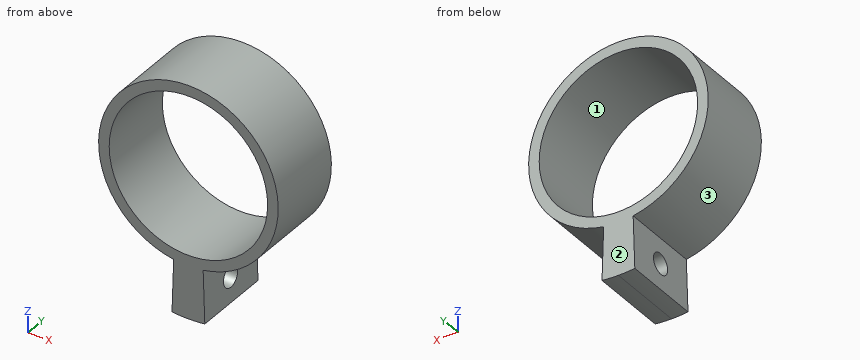
from build123d import *

# Parameters (mm, degrees)
F0_R     = 17
F0_R_2   = 15
F1_DEPTH = 15
F3_DEPTH = 15
F4_R     = 2
F5_DEPTH = 20.10135


with BuildPart() as f1:
    # F0 (on Front) → F1 (new body)
    with BuildSketch(Plane.XZ):
        Circle(F0_R)
        Circle(F0_R_2, mode=Mode.SUBTRACT)
    extrude(amount=F1_DEPTH)

    # F2 (on face) → F3 (join)
    with BuildSketch(Plane(origin=(0, 0, 0), x_dir=(-1, 0, 0), z_dir=(0, 1, 0))):
        with BuildLine():
            Line((-2.790576, -16.769397), (-3.104631, -26.764465))
            ThreePointArc((-3.104631, -26.764465), (-1.554907, -26.899025), (0, -26.943929))
            ThreePointArc((0, -26.943929), (1.554907, -26.899025), (3.104631, -26.764465))
            Line((3.104631, -26.764465), (2.790576, -16.769397))
            ThreePointArc((2.790576, -16.769397), (1.400044, -16.942251), (0, -17))
            ThreePointArc((0, -17), (-1.400044, -16.942251), (-2.790576, -16.769397))
        make_face()
    extrude(amount=-F3_DEPTH)

    # F4 (on face) → F5 (cut, through all)
    with BuildSketch(Plane(origin=(-2.261431, 0, 0.071057), x_dir=(0, -1, 0), z_dir=(-0.999507, 0, 0.031406))):
        with Locations((7.5, -21.848765)):
            Circle(F4_R)
    extrude(amount=-F5_DEPTH, mode=Mode.SUBTRACT)


solid = f1.part
Design review of the part built by this model. Coordinates are the model's own, in mm. Face numbers are marked on the shaded views. Round coordinates to 2 decimals unless told otherwise and drop trailing zeros. Write each loop counter-clockwise with the first axis right and the second up, starting at its lowest first coordinate (ties: lowest second). Pieces come first, ordered by that corner, then holes. Notation, with made-up numbers: (19.5, 85.5) -> (71.5, 85.5) arc R26 ccw to (71.5, 120.5) -> close; hole circle Ø6 at (83, -19.75). An arc over 180 degrees is marked (long way). One line per question, with ' | ' between items.
(1) Take a section at D-D, the plane y = -3.25. State the section outline as (x, z) points.
Result sheet:
outline: (-3.1, -26.76) arc R26.94 ccw to (0, -26.94) arc R26.94 ccw to (3.1, -26.76) -> (2.79, -16.77) arc R17 ccw (long way) to (-2.79, -16.77) -> close; hole circle Ø30 at (0, 0)
(2) Take a section at A-A, the plane z = 0. State the section outline as (x, y) points.
Result sheet:
outline: (-17, -15) -> (-15, -15) -> (-15, 0) -> (-17, 0) -> close; (15, -15) -> (17, -15) -> (17, 0) -> (15, 0) -> close
(3) Insertion check: P1, Ø5, axis at y = -7, z = -4.5, coming from the +X side; P2, Ø6, axis at y = -6, z = 1, coming from the -X side; P3, Ø8, axis at x = -8.5, y = -11.5, coming from the +Z side; P4, Ø6, axis at x = 11, y = -12, coming from the -Z side. Each pin has a flat end and moves straight along its axis. Give the tip position at first contact, or say it passes through.
Result sheet:
P1: x = 16.88 | P2: x = -17 | P3: z = 16.39 | P4: z = -15
(4) Take a section at B-B, the plane y = -6.5. State the section outline as (x, z) points, and give its area (3 significant figures).
Result sheet:
outline: (-3.1, -26.76) arc R26.94 ccw to (0, -26.94) arc R26.94 ccw to (3.1, -26.76) -> (3.01, -23.69) -> (-3, -23.5) -> close; (-2.89, -20.04) -> (2.9, -20.22) -> (2.79, -16.77) arc R17 ccw (long way) to (-2.79, -16.77) -> close; hole circle Ø30 at (0, 0) | area: 239 mm2
(5) Draft analysis for pull direction X (two halves, no side actions). For the marked faces 1, 2 and 3, state which applies: released by +X, released by -X, zero draft, split by the parting line, or undercut.
Result sheet:
face 1: undercut | face 2: zero draft | face 3: split by the parting line
(6) Wall thickness on line 1 (Z direction, x = 0, y = -3.75); line 2 (Z direction, x = 0, y = -8); line 3 (Z direction, x = -2, y = -9): over which ranges is each line inside the solid? List them lowest first. Write a range as [from, to].
Result sheet:
line 1: [-26.94, -15], [15, 17] | line 2: [-26.94, -23.8], [-19.92, -15], [15, 17] | line 3: [-26.87, -23.12], [-20.47, -14.87], [14.87, 16.88]
(7) Take a section at C-C, the plane x = 11. State the section outline as (y, z) points.
Result sheet:
outline: (-15, -12.96) -> (0, -12.96) -> (0, -10.2) -> (-15, -10.2) -> close; (-15, 10.2) -> (0, 10.2) -> (0, 12.96) -> (-15, 12.96) -> close
